Check sheet for the modelled part. Datum: model origin and axes. Units: mm. A direction names the side the tool comes from. Give positions to 0.01 mm unless a question says otherwise; leave off trailing zeros. Order: outer loops, then holes, each group sorted by start corner. A loop starts at its lowest first (then second) coordinate and runs counter-clockwise, first axis right, second up. Notation, with made-up numbers: (-28, 22.5) - (24, 22.5) arc R29 ccw to (24, 44.5) - close; hole circle Ø10 at (-11.5, 72). An arc over 180 degrees is marked (long way). Answer in a Markdown table with one row per item.
from build123d import *

# Parameters (mm, degrees)
SKETCH1_R           = 21.8
SKETCH1_R_2         = 16.8
BOSS_EXTRUDE1_DEPTH = 80
SKETCH3_R           = 21.8
BOSS_EXTRUDE2_DEPTH = 1
SKETCH4_R           = 12.7
BOSS_EXTRUDE3_DEPTH = 8


with BuildPart() as part:
    # Sketch1 → Boss-Extrude1 (new body)
    with BuildSketch(Plane(origin=(0, 0, 0), x_dir=(1, 0, 0), z_dir=(0, 1, 0))):
        Circle(SKETCH1_R)
        Circle(SKETCH1_R_2, mode=Mode.SUBTRACT)
    extrude(amount=BOSS_EXTRUDE1_DEPTH)

    # Sketch3 → Boss-Extrude2 (add)
    with BuildSketch(Plane(origin=(0, 80, 0), x_dir=(1, 0, 0), z_dir=(0, 1, 0))):
        Circle(SKETCH3_R)
    extrude(amount=BOSS_EXTRUDE2_DEPTH)

    # Sketch4 → Boss-Extrude3 (add)
    with BuildSketch(Plane(origin=(0, 81, 0), x_dir=(1, 0, 0), z_dir=(0, 1, 0))):
        Circle(SKETCH4_R)
    extrude(amount=BOSS_EXTRUDE3_DEPTH)


solid = part.part
(1) Access from +Z, -Z, +X, -X, +Y, -Y to the whole of each face (thin tool, end or side, straight path). Record for faces 4 (the flat face through (0, 80, 0)), 5 (the flat face through (9.4, 81, 9.4)), 6 (the cylindrical face through (20.793, 39.933, -6.548)).
Geometry says:
| item | result |
|---|---|
| face 4 | -Y |
| face 5 | +Y |
| face 6 | +Y, -Y |
(2) Cross-section at B-B, the plane z = 0. Record the cut outline in (x, y).
Geometry says:
| item | result |
|---|---|
| outline | (-21.8, 0) - (-16.8, 0) - (-16.8, 80) - (16.8, 80) - (16.8, 0) - (21.8, 0) - (21.8, 81) - (12.7, 81) - (12.7, 89) - (-12.7, 89) - (-12.7, 81) - (-21.8, 81) - close |
(3) Thickness scan on L1, parallel to Z at x = 0, y = 25; L2, parallel to Y at x = -6, z = 16.5. Record the ranges inside material, lowest first.
Geometry says:
| item | result |
|---|---|
| L1 | -21.8 to -16.8, 16.8 to 21.8 |
| L2 | 0 to 81 |
(4) Cross-section at C-C, the plane y = 32. Record the cut outline in (x, z), then the cut area to 3 significant figures.
Geometry says:
| item | result |
|---|---|
| outline | circle Ø43.6 at (0, 0); hole circle Ø33.6 at (0, 0) |
| area | 606 mm² |
(5) Cross-section at D-D, the plane y = 83. Record the cut outline in (x, z).
Geometry says:
| item | result |
|---|---|
| outline | circle Ø25.4 at (0, 0) |
(6) Cross-section at A-A, the plane x = 0. Record the cut outline in (y, z).
Geometry says:
| item | result |
|---|---|
| outline | (0, -21.8) - (81, -21.8) - (81, -12.7) - (89, -12.7) - (89, 12.7) - (81, 12.7) - (81, 21.8) - (0, 21.8) - (0, 16.8) - (80, 16.8) - (80, -16.8) - (0, -16.8) - close |
(7) Gauge pin test, flat ends, axial feed: P1, Ø2, axis at x = -0.5, y = 80, coming from the -Z side; P2, Ø1, axis at y = 75.5, z = -12, coming from the +X side; P3, Ø10, axis at y = 65, z = 11.5, coming from the +X side. Record the tip position at first contact, or that the pin passes through.
Geometry says:
| item | result |
|---|---|
| P1 | z = -21.8 |
| P2 | x = 18.52 |
| P3 | x = 20.81 |
(8) Mould release check, pull along Z, two halves, no side actions. Record for faces 1 (the cylindrical face through (-2.75, 84.94, 12.4)), 2 (the flat face through (0, 89, 0)), 3 (the cylindrical face through (16.024, 39.44, -5.046)): pulls with the +Z half, pulls with the -Z half, needs draft (parallel to the pull), parting line crosses it, or undercut.
Geometry says:
| item | result |
|---|---|
| face 1 | parting line crosses it |
| face 2 | needs draft |
| face 3 | undercut |
